Autodesk Inventor part; units mm, degrees
ref_plane "YZ Plane" through (0, 0, 0) normal (1, 0, 0) x (0, 1, 0)
ref_plane "XZ Plane" through (0, 0, 0) normal (0, 1, 0) x (-1, 0, 0)
ref_plane "XY Plane" through (0, 0, 0) normal (0, 0, 1) x (1, 0, 0)
sketch "Sketch1" plane through (0, 0, 0) normal (0, 0, 1) x (1, 0, 0)
  line L0 (0, 0) -> (1104.9, 0)
  line L1 (1104.9, 0) -> (1104.9, 203.2)
  line L2 (1104.9, 203.2) -> (0, 203.2)
  line L3 (0, 203.2) -> (0, 0)
  dimension "d0" = 1104.9
  dimension "d1" = 203.2
extrude "Extrusion1" add sketch "Sketch1" along normal blind 20.32
sketch "Sketch2" plane through (0, 0, 20.32) normal (0, 0, 1) x (1, 0, 0)
  line L0 (1104.9, 0) -> (1104.9, 203.2)
  line L1 (0, 0) -> (1104.9, 0)
  line L2 (1104.9, 57.15) -> (723.9, 57.15)
  line L3 (723.9, 57.15) -> (723.9, 0)
  line L4 (723.9, 0) -> (1104.9, 0)
  line L5 (1104.9, 0) -> (1104.9, 57.15)
  line L6 (723.9, 0) -> (629.2025, 135.242)
  line L7 (723.9, 0) -> (671.9967, -36.3431)
  line L8 (629.2025, 135.242) -> (585.2084, 160.642)
  line L9 (585.2084, 160.642) -> (407.4084, 145.0865)
  line L10 (787.4, 57.15) -> (731.14, 177.8)
  line L11 (731.14, 177.8) -> (676.6695, 203.2)
  line L12 (1104.9, 203.2) -> (0, 203.2)
  line L13 (676.6695, 203.2) -> (407.4084, 179.6427)
  line L14 (787.4, 57.15) -> (723.9, 57.15)
  line L15 (723.9, 57.15) -> (723.9, 0)
  line L16 (407.4084, 179.6427) -> (0, 27.5632)
  line L17 (407.4084, 145.0865) -> (26.4084, 2.8648)
  line L18 (0, 203.2) -> (0, 0)
  line L19 (26.4084, 2.8648) -> (0, 27.5632)
  line L20 (407.4084, 145.0865) -> (365.4136, 141.4124)
  dimension "d4" = 57.15
  dimension "d5" = 381
  dimension "d6" = 125
  dimension "d7" = 165.1
  dimension "d8" = 50.8
  dimension "d9" = 155
  dimension "d10" = 145
  dimension "d11" = 177.8
  dimension "d12" = 317.5
  dimension "d13" = 115
  dimension "d14" = 120.65
  dimension "d15" = 140
  dimension "d16" = 0
  dimension "d18" = 381
  dimension "d19" = 0
  dimension "d33" = 15.47
extrude "Extrusion2" cut sketch "Sketch2" against normal blind 20.32 contours L2 L10 L11 L12 L0 | L1 L18 L19 L17 L9 L8 L6 | L13 L16 L18 L12
fillet "Fillet1" radius 28.575 2 edges at (1104.9, 0, 10.16) (1104.9, 57.15, 10.16)
fillet "Fillet2" radius 57.15 1 edges at (723.9, 0, 10.16)
fillet "Fillet3" radius 6.35 3 edges at (629.2025, 135.242, 10.16) (585.2084, 160.642, 10.16) (407.4084, 145.0865, 10.16)
fillet "Fillet4" radius 25.4 3 edges at (676.6695, 203.2, 10.16) (731.14, 177.8, 10.16) (407.4084, 179.6427, 10.16)
sketch "Sketch3" plane through (0, 0, 0) normal (0, 0, -1) x (-1, 0, 0)
  circle A0 centre (-1076.325, 28.575) radius 6.35
  line L0 (-753.6504, 0) -> (-1076.325, 0)
  arc A1 (-1076.325, 57.15) -> (-1076.325, 0) centre (-1076.325, 28.575) ccw
  point P0 (0, 0)
  dimension "d26" = 12.7
  dimension "d29" = 0
  dimension "d30" = 0
extrude "Extrusion3" cut sketch "Sketch3" against normal blind 20.32
properties part number "Kermit Mount"
Work out the finished part from the listing and answer in its coordinate system (mm). A direction names the side the tool comes from. Round coordinates to 2 decimals unless told otherwise and drop trailing zeros. Write each loop counter-clockwise with the first axis right and the second up, starting at its lowest first coordinate (ties: lowest second). Pieces come first, ordered by that corner, then holes. Notation, with made-up numbers: (22, 25) -> (55, 25) arc R26 cw to (55, 54) -> close; hole circle Ø9 at (67, 88.25). An arc over 180 degrees is marked (long way). Answer as CSV lines item,"result". Start each with the question number.
(1) The mould has two halves that part along X. Classify faces 4 (the flat face through (496.965, 152.922, 10.302)), 5 (the flat face through (673, 87, 0)), 6 (the cylindrical face through (1096.31, 49, 10.02)): +X half, -X half, draft (parallel to the pull), parting line (faces both ways), or undercut.
(2) The part is cut by section A-A, the plane y = 113.5. Give the vertices of the cut face in (x, z).
(3) The part is cut by section D-D, the plane x = 264.5. Give the vertices of the cut face in (y, z), then the cut area to 3 significant figures.
(4) The part is cut by section C-C, the plane x = 905.5. Give the vertices of the cut face in (y, z), then the cut area to 3 significant figures.
(5) A tool of negligible diameter and unlimited length cuts with its end or side. For faces 1 (the flat face through (13.39, 15.04, 10.3)), 2 (the cylindrical face through (727.603, 6.281, 10.018)), 3 (the flat face through (934, 57.15, 10)), from which of +Z, -Z, +X, -X, +Y, -Y can it reach the whole face along a straight path? Write none if from no direction.
(6) Each of these flat-tipped pins is pushed along its axis until it touches: pin 1 (6 mm diameter, centred on x = 931, z = 7, fed in from +Y); pin 2 (2 mm diameter, centred on x = 419, z = 6.5, fed in from -Y); pin 3 (12 mm diameter, centred on y = 117, z = 2.5, fed in from +X). Where does it stop, or does it pass through?
(7) Find the intervals of material crossed by probe 1 along Y at (x, z) = (880.5, 9.5); probe 2 along Y at (x, z) = (414, 16.5), in increasing order.
Output values:
1,face 4,"undercut"
1,face 5,"draft"
1,face 6,"+X half"
2,outline,"(230.22, 0) -> (322.79, 0) -> (322.79, 20.32) -> (230.22, 20.32) -> close; (644.43, 0) -> (761.12, 0) -> (761.12, 20.32) -> (644.43, 20.32) -> close"
3,outline,"(91.74, 0) -> (126.3, 0) -> (126.3, 20.32) -> (91.74, 20.32) -> close"
3,area,"702 mm²"
4,outline,"(0, 0) -> (57.15, 0) -> (57.15, 20.32) -> (0, 20.32) -> close"
4,area,"1,160 mm²"
5,face 1,"+Z, -Z, -X, -Y"
5,face 2,"+Z, -Z, -Y"
5,face 3,"+Z, -Z, +X, +Y"
6,pin 1,"stops at y = 57.15"
6,pin 2,"stops at y = 146.01"
6,pin 3,"stops at x = 762.29"
7,probe 1,"y = 0 to 57.15"
7,probe 2,"y = 145.66 to 180.22"
